Geometry check sheet. Reference: the model listing, model coordinates, mm. Round coordinates to 2 decimals unless told otherwise and drop trailing zeros. Write each loop counter-clockwise with the first axis right and the second up, starting at its lowest first coordinate (ties: lowest second). Pieces come first, ordered by that corner, then holes. Notation, with made-up numbers: (18.5, -22.75) -> (39.5, -22.75) arc R28 ccw to (39.5, -1.75) -> close; hole circle Ø3 at (-1.5, 14). An arc over 180 degrees is marked (long way). Put each result on its own line as item: value. Start each with the question number.
from build123d import *

# Parameters (mm, degrees)
F1_DEPTH = 6.35
F2_SIZE  = 2.54
F3_SIZE  = 2.54


with BuildPart() as f1:
    # F0 (on Front) → F1 (new body)
    with BuildSketch(Plane.XZ):
        Polygon((101.6, 101.6), (0, 0), (101.6, 0), align=None)
    extrude(amount=F1_DEPTH)

    # F2
    f2_edges = [f1.edges().sort_by_distance(p)[0] for p in [
        (101.6, -6.35, 50.8),
        (50.8, -6.35, 0),
    ]]
    chamfer(f2_edges, length=F2_SIZE)

    # F3
    f3_edges = [f1.edges().sort_by_distance(p)[0] for p in [
        (101.6, 0, 50.8),
        (50.8, 0, 0),
    ]]
    chamfer(f3_edges, length=F3_SIZE)


solid = f1.part
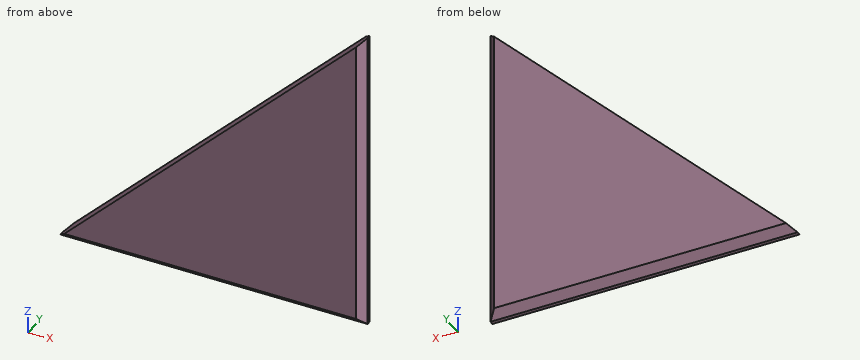
(1) Sectioned sample at B-B (z = 48.5). Record the cut outline in (x, y), and give its area (3 significant figures).
(2) Sectioned sample at A-A (x = 86). Record the cut outline in (y, z), and give its area (3 significant figures).
(3) Go/stop test with flat-tipped pins: pin 1 Ø3 at (y, z) = (-2, 20.5) entering from +X; pin 2 Ø1 at (x, y) = (50, -3) entering from +Z. Record where each tip stops, or that it passes through.
(4) Material ranges on L1, parallel to X at y = -1.75, z = 77.5; L2, parallel to Z at x = 17, y = -0.25; L3, parallel to X at y = -2.25, z = 76.5, recorded low to high. Write a range as from..to.
(5) Sectioned sample at C-C (y = -5). Record the cut outline in (x, z).
Found:
1. outline: (48.5, -6.35) -> (99.06, -6.35) -> (101.6, -3.81) -> (101.6, -2.54) -> (99.06, 0) -> (48.5, 0) -> close
1. area: 331 mm2
2. outline: (-6.35, 2.54) -> (-3.81, 0) -> (-2.54, 0) -> (0, 2.54) -> (0, 86) -> (-6.35, 86) -> close
2. area: 540 mm2
3. pin 1: x = 101.6
3. pin 2: z = 50.5
4. L1: 77.5..100.81
4. L2: 2.29..17
4. L3: 76.5..101.31
5. outline: (1.19, 1.19) -> (100.41, 1.19) -> (100.41, 100.41) -> close
